```python
from build123d import *

# Parameters (mm, degrees)
ESQUISSE1_R        = 2.5
BOSS_EXTRU_1_DEPTH = 3


with BuildPart() as part:
    # Esquisse1 → Boss.-Extru.1 (new body)
    with BuildSketch(Plane.XY.offset(3)):
        Polygon((83.180673727, 37.513816477), (68.04858861, 52.645901594), (65.715136232, 50.312449216), (62.055338257, 53.972247191), (-2.441299609, 53.972247191), (-6.101097584, 50.312449216), (-8.434549962, 52.645901594), (-23.566635079, 37.513816477), (-21.233182701, 35.180364099), (-24.892980676, 31.520566124), (-24.892980676, -32.976071742), (-21.233182701, -36.635869717), (-23.566635079, -38.969322095), (-8.434549962, -54.101407212), (-6.101097584, -51.767954834), (-2.441299609, -55.427752809), (62.055338257, -55.427752809), (65.715136232, -51.767954834), (68.04858861, -54.101407212), (83.180673727, -38.969322095), (80.847221349, -36.635869717), (84.507019324, -32.976071742), (84.507019324, 31.520566124), (80.847221349, 35.180364099), align=None)
        with Locations((-10.131606237, 39.210872752)):
            Circle(ESQUISSE1_R, mode=Mode.SUBTRACT)
        with Locations((69.745644885, -40.66637837)):
            Circle(ESQUISSE1_R, mode=Mode.SUBTRACT)
    extrude(amount=-BOSS_EXTRU_1_DEPTH)


solid = part.part
```
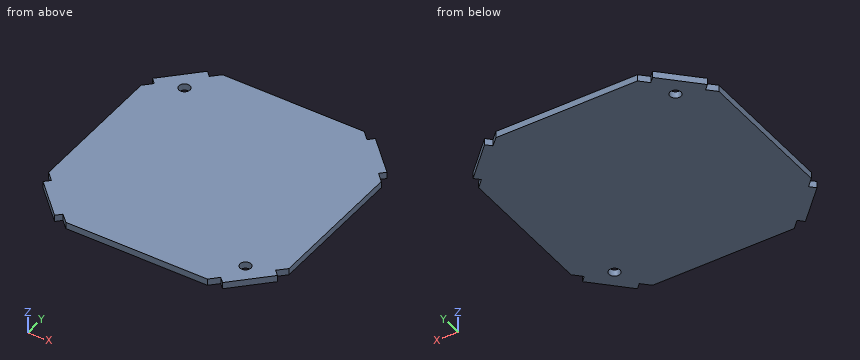
For this review, take the finished solid that the model builds, in its own axes (mm). Round coordinates to 2 decimals unless told otherwise and drop trailing zeros. Write each loop counter-clockwise with the first axis right and the second up, starting at its lowest first coordinate (ties: lowest second). Pieces come first, ordered by that corner, then holes.
1) Take a section at C-C on x = 77. Give the boundary of the cut face in (y, z), then the cut area to 3 significant figures.
Answer below:
outline: (-45.15, 0) - (43.69, 0) - (43.69, 3) - (-45.15, 3) - close
area: 267 mm2
2) Take a section at B-B on z = 2.1. Give the boundary of the cut face in (x, y), then the cut area to 3 significant figures.
Answer below:
outline: (-24.89, -32.98) - (-21.23, -36.64) - (-23.57, -38.97) - (-8.43, -54.1) - (-6.1, -51.77) - (-2.44, -55.43) - (62.06, -55.43) - (65.72, -51.77) - (68.05, -54.1) - (83.18, -38.97) - (80.85, -36.64) - (84.51, -32.98) - (84.51, 31.52) - (80.85, 35.18) - (83.18, 37.51) - (68.05, 52.65) - (65.72, 50.31) - (62.06, 53.97) - (-2.44, 53.97) - (-6.1, 50.31) - (-8.43, 52.65) - (-23.57, 37.51) - (-21.23, 35.18) - (-24.89, 31.52) - close; hole circle Ø5 at (-10.13, 39.21); hole circle Ø5 at (69.75, -40.67)
area: 11,200 mm2
3) Insertion check: pin 1 Ø6 at (x, y) = (68.5, 3.5) entering from -Z. The pin has a flat end and moves straight along its axis. Give the tip position at first contact, or say it passes through.
Answer below:
pin 1: stops at z = 0
4) Take a section at A-A on x = -11. Give the boundary of the cut face in (y, z), then the cut area to 3 significant figures.
Answer below:
outline: (-51.54, 0) - (36.87, 0) - (36.87, 3) - (-51.54, 3) - close; (41.56, 0) - (50.08, 0) - (50.08, 3) - (41.56, 3) - close
area: 291 mm2
5) For line 1 along Y through (x, z) = (-11, 1.7); line 2 along Y through (x, z) = (67.5, 1.6); line 3 along X through (y, z) = (-44.5, 1.65), list the stretches that pass through material, from the lowest coordinate up.
Answer below:
line 1: y = -51.54 to 36.87, 41.56 to 50.08
line 2: y = -53.55 to -41.77, -39.57 to 52.1
line 3: x = -18.04 to 77.65
